Geometry: final body of the model. Coordinates: model frame, mm. Give positions to 0.01 mm unless a question says otherwise; leave off trailing zeros. Order: outer loops, then holes, each group sorted by start corner. A loop starts at its lowest first (then second) coordinate and runs counter-clockwise, first axis right, second up. Notation, with made-up numbers: (47, 61.5) -> (88, 61.5) arc R35 ccw to (88, 100.5) -> close; hole circle Ø2 at (80.5, 53.5). An arc over 180 degrees is marked (long way). One line per question, with ' | ' between items.
from build123d import *

# Parameters (mm, degrees)
ESQUISSE1_W               = 482.6
ESQUISSE1_H               = 177.8
T_LE_DE_BASE_PLI_E1_DEPTH = 3.03784
ENL_V_MAT_EXTRU_1_DEPTH   = 258.173343237
CONG_1_R                  = 2.54
ESQUISSE5_R               = 58.42
ENL_V_MAT_EXTRU_2_DEPTH   = 258.173343237
ESQUISSE6_R               = 2.1844
ENL_V_MAT_EXTRU_3_DEPTH   = 258.173343237
ESQUISSE7_R               = 3.317875
ENL_V_MAT_EXTRU_4_DEPTH   = 258.173343237


# Sheet-metal steps are written as plain solids
with BuildPart() as part:
    # Esquisse1 → Tôle de base pliée1 (new body)
    with BuildSketch(Plane.XY):
        Rectangle(ESQUISSE1_W, ESQUISSE1_H)
    extrude(amount=-T_LE_DE_BASE_PLI_E1_DEPTH)

    # Esquisse4 → Enlèv. mat.-Extru.1 (cut, through all)
    with BuildSketch(Plane.XY):
        with BuildLine():
            Line((-234.536234, -78.978125), (-231.361234, -78.978125))
            ThreePointArc((-231.361234, -78.978125), (-227.789359, -82.55), (-231.361234, -86.121875))
            Line((-231.361234, -86.121875), (-234.536234, -86.121875))
            ThreePointArc((-234.536234, -86.121875), (-238.108109, -82.55), (-234.536234, -78.978125))
        make_face()
        with BuildLine():
            Line((-234.536234, 86.121875), (-231.361234, 86.121875))
            ThreePointArc((-231.361234, 86.121875), (-227.789359, 82.55), (-231.361234, 78.978125))
            Line((-231.361234, 78.978125), (-234.536234, 78.978125))
            ThreePointArc((-234.536234, 78.978125), (-238.108109, 82.55), (-234.536234, 86.121875))
        make_face()
        with BuildLine():
            Line((231.361234, 86.121875), (234.536234, 86.121875))
            ThreePointArc((234.536234, 86.121875), (238.108109, 82.55), (234.536234, 78.978125))
            Line((234.536234, 78.978125), (231.361234, 78.978125))
            ThreePointArc((231.361234, 78.978125), (227.789359, 82.55), (231.361234, 86.121875))
        make_face()
        with BuildLine():
            Line((231.361234, -78.978125), (234.536234, -78.978125))
            ThreePointArc((234.536234, -78.978125), (238.108109, -82.55), (234.536234, -86.121875))
            Line((234.536234, -86.121875), (231.361234, -86.121875))
            ThreePointArc((231.361234, -86.121875), (227.789359, -82.55), (231.361234, -78.978125))
        make_face()
        with BuildLine():
            Line((-234.536234, -34.528125), (-231.361234, -34.528125))
            ThreePointArc((-231.361234, -34.528125), (-227.789359, -38.1), (-231.361234, -41.671875))
            Line((-231.361234, -41.671875), (-234.536234, -41.671875))
            ThreePointArc((-234.536234, -41.671875), (-238.108109, -38.1), (-234.536234, -34.528125))
        make_face()
        with BuildLine():
            Line((-234.536234, -47.228125), (-231.361234, -47.228125))
            ThreePointArc((-231.361234, -47.228125), (-227.789359, -50.8), (-231.361234, -54.371875))
            Line((-231.361234, -54.371875), (-234.536234, -54.371875))
            ThreePointArc((-234.536234, -54.371875), (-238.108109, -50.8), (-234.536234, -47.228125))
        make_face()
        with BuildLine():
            Line((231.361234, -47.228125), (234.536234, -47.228125))
            ThreePointArc((234.536234, -47.228125), (238.108109, -50.8), (234.536234, -54.371875))
            Line((234.536234, -54.371875), (231.361234, -54.371875))
            ThreePointArc((231.361234, -54.371875), (227.789359, -50.8), (231.361234, -47.228125))
        make_face()
        with BuildLine():
            Line((231.361234, -34.528125), (234.536234, -34.528125))
            ThreePointArc((234.536234, -34.528125), (238.108109, -38.1), (234.536234, -41.671875))
            Line((234.536234, -41.671875), (231.361234, -41.671875))
            ThreePointArc((231.361234, -41.671875), (227.789359, -38.1), (231.361234, -34.528125))
        make_face()
        with BuildLine():
            Line((-234.536234, 9.921875), (-231.361234, 9.921875))
            ThreePointArc((-231.361234, 9.921875), (-227.789359, 6.35), (-231.361234, 2.778125))
            Line((-231.361234, 2.778125), (-234.536234, 2.778125))
            ThreePointArc((-234.536234, 2.778125), (-238.108109, 6.35), (-234.536234, 9.921875))
        make_face()
        with BuildLine():
            Line((-234.536234, -2.778125), (-231.361234, -2.778125))
            ThreePointArc((-231.361234, -2.778125), (-227.789359, -6.35), (-231.361234, -9.921875))
            Line((-231.361234, -9.921875), (-234.536234, -9.921875))
            ThreePointArc((-234.536234, -9.921875), (-238.108109, -6.35), (-234.536234, -2.778125))
        make_face()
        with BuildLine():
            Line((231.361234, 54.371875), (234.536234, 54.371875))
            ThreePointArc((234.536234, 54.371875), (238.108109, 50.8), (234.536234, 47.228125))
            Line((234.536234, 47.228125), (231.361234, 47.228125))
            ThreePointArc((231.361234, 47.228125), (227.789359, 50.8), (231.361234, 54.371875))
        make_face()
        with BuildLine():
            Line((231.361234, 41.671875), (234.536234, 41.671875))
            ThreePointArc((234.536234, 41.671875), (238.108109, 38.1), (234.536234, 34.528125))
            Line((234.536234, 34.528125), (231.361234, 34.528125))
            ThreePointArc((231.361234, 34.528125), (227.789359, 38.1), (231.361234, 41.671875))
        make_face()
        with BuildLine():
            Line((-234.536234, 54.371875), (-231.361234, 54.371875))
            ThreePointArc((-231.361234, 54.371875), (-227.789359, 50.8), (-231.361234, 47.228125))
            Line((-231.361234, 47.228125), (-234.536234, 47.228125))
            ThreePointArc((-234.536234, 47.228125), (-238.108109, 50.8), (-234.536234, 54.371875))
        make_face()
        with BuildLine():
            Line((-234.536234, 41.671875), (-231.361234, 41.671875))
            ThreePointArc((-231.361234, 41.671875), (-227.789359, 38.1), (-231.361234, 34.528125))
            Line((-231.361234, 34.528125), (-234.536234, 34.528125))
            ThreePointArc((-234.536234, 34.528125), (-238.108109, 38.1), (-234.536234, 41.671875))
        make_face()
        with BuildLine():
            Line((231.361234, 9.921875), (234.536234, 9.921875))
            ThreePointArc((234.536234, 9.921875), (238.108109, 6.35), (234.536234, 2.778125))
            Line((234.536234, 2.778125), (231.361234, 2.778125))
            ThreePointArc((231.361234, 2.778125), (227.789359, 6.35), (231.361234, 9.921875))
        make_face()
        with BuildLine():
            Line((231.361234, -2.778125), (234.536234, -2.778125))
            ThreePointArc((234.536234, -2.778125), (238.108109, -6.35), (234.536234, -9.921875))
            Line((234.536234, -9.921875), (231.361234, -9.921875))
            ThreePointArc((231.361234, -9.921875), (227.789359, -6.35), (231.361234, -2.778125))
        make_face()
    extrude(amount=-ENL_V_MAT_EXTRU_1_DEPTH, mode=Mode.SUBTRACT)

    # Congé1
    cong_1_edges = [part.edges().sort_by_distance(p)[0] for p in [
        (-241.3, 88.9, -1.51892),
        (241.3, 88.9, -1.51892),
        (241.3, -88.9, -1.51892),
        (-241.3, -88.9, -1.51892),
    ]]
    fillet(cong_1_edges, radius=CONG_1_R)

    # Esquisse5 → Enlèv. mat.-Extru.2 (cut, through all)
    with BuildSketch(Plane.XY):
        Circle(ESQUISSE5_R)
        with Locations((-139.7, 0)):
            Circle(ESQUISSE5_R)
        with Locations((139.7, 0)):
            Circle(ESQUISSE5_R)
    extrude(amount=-ENL_V_MAT_EXTRU_2_DEPTH, mode=Mode.SUBTRACT)

    # Esquisse6 → Enlèv. mat.-Extru.3 (cut, through all)
    with BuildSketch(Plane(origin=(0, 0, -3.03784), x_dir=(-1, 0, 0), z_dir=(0, 0, -1))):
        with Locations((-192.2, 52.5)):
            Circle(ESQUISSE6_R)
        with Locations((-87.2, 52.5)):
            Circle(ESQUISSE6_R)
        with Locations((-52.5, 52.5)):
            Circle(ESQUISSE6_R)
        with Locations((-87.2, -52.5)):
            Circle(ESQUISSE6_R)
        with Locations((-52.5, -52.5)):
            Circle(ESQUISSE6_R)
        with Locations((-192.2, -52.5)):
            Circle(ESQUISSE6_R)
        with Locations((52.5, 52.5)):
            Circle(ESQUISSE6_R)
        with Locations((52.5, -52.5)):
            Circle(ESQUISSE6_R)
        with Locations((87.2, -52.5)):
            Circle(ESQUISSE6_R)
        with Locations((87.2, 52.5)):
            Circle(ESQUISSE6_R)
        with Locations((192.2, 52.5)):
            Circle(ESQUISSE6_R)
        with Locations((192.2, -52.5)):
            Circle(ESQUISSE6_R)
    extrude(amount=-ENL_V_MAT_EXTRU_3_DEPTH, mode=Mode.SUBTRACT)

    # Esquisse7 → Enlèv. mat.-Extru.4 (cut, through all)
    with BuildSketch(Plane.XY):
        with Locations((-203.2, 76.2)):
            Circle(ESQUISSE7_R)
        with Locations((-203.2, -76.2)):
            Circle(ESQUISSE7_R)
        with Locations((203.2, -76.2)):
            Circle(ESQUISSE7_R)
        with Locations((203.2, 76.2)):
            Circle(ESQUISSE7_R)
    extrude(amount=-ENL_V_MAT_EXTRU_4_DEPTH, mode=Mode.SUBTRACT)


solid = part.part
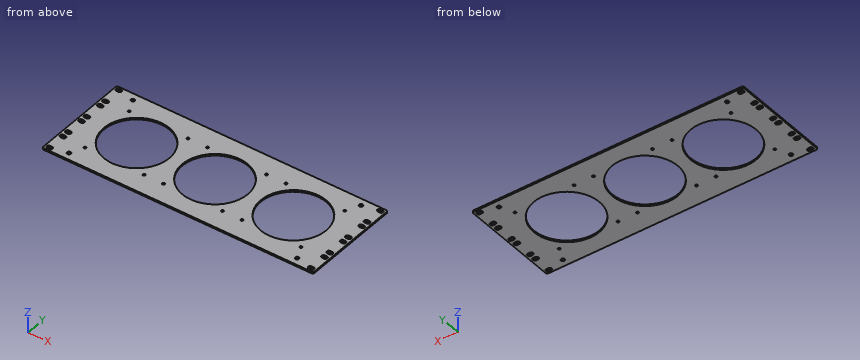
1) Section C-C on x = 117. Return loops of the section in (y, z).
Check result:
outline: (-88.9, -3.04) -> (-53.83, -3.04) -> (-53.83, 0) -> (-88.9, 0) -> close; (53.83, -3.04) -> (88.9, -3.04) -> (88.9, 0) -> (53.83, 0) -> close
2) Contact query for a flat-ended pin moving along its axis: pin 1 Ø3.5 at (x, y) = (192.2, 52.5) entering from -Z. Output: stop coordinate, or through.
Check result:
pin 1: passes through
3) Material intervals for probe 1 along X at (y, z) = (2, -1); probe 2 along Y at (x, z) = (-192.2, -1.75); probe 3 along X at (y, z) = (-50, -0.7), sorted ascending. Write a range as from..to.
Check result:
probe 1: x = -241.3..-198.09, -81.31..-58.39, 58.39..81.31, 198.09..241.3 | probe 2: y = -88.9..-54.68, -50.32..-25.63, 25.63..50.32, 54.68..88.9 | probe 3: x = -241.3..-238.02, -227.88..-169.91, -109.49..-30.21, 30.21..109.49, 169.91..227.88, 238.02..241.3
4) Section A-A on x = -139.7. Return loops of the section in (y, z).
Check result:
outline: (-88.9, -3.04) -> (-58.42, -3.04) -> (-58.42, 0) -> (-88.9, 0) -> close; (58.42, -3.04) -> (88.9, -3.04) -> (88.9, 0) -> (58.42, 0) -> close
5) Section B-B on z = -1.4. Count the separate pieces of the cut face and the enclosed holes in it, plus the area to 3 significant figures.
Check result:
separate pieces: 1 | enclosed holes: 35 | area: 52,300 mm^2
